Could you check a few things on this drawing? It's one solid part, dimensions in mm from its lowest x, y, z. A direction names the side the tool comes from. Give positions to 0.01 mm unless a question says otherwise; leave off trailing zeros. Order: outer loops, then holes, each group sorted by start corner. A loop starts at its lowest first (then second) coordinate and runs counter-clockwise, first axis right, second up. Notation, with made-up numbers: M 68,17.25 L 111,17.25 A25 cw 111,50.25 Z; hole C 67,80 d5. An arc over 180 degrees is marked long. Use one line per item in the form item = value. Start each with the question number.
1. I want a section at D-D, the plane x = 8.25. List the corners of the cut face in (y, z) for me, and give its area (3 significant figures).
2. Will these pins go through, and if not, where does the flat tip stop? P1, Ø3, axis at x = 6.5, y = 4, coming from the +Z side; P2, Ø4, axis at x = 7, z = 8, coming from the -Y side.
3. I want a section at A-A, the plane z = 6.5. List the corners of the cut face in (x, y) for me.
4. For the marked faces 4, 5, 6, 7 and 8, which set-ups out of +Z, -Z, +X, -X, +Y, -Y let a thin tool reach every point of the face, with its end or its side?
5. We'd pull the mould along Z, two halves only. Please class the marked faces 1, 2 and 3: +Z half, -Z half, draft (parallel to the pull), parting line (faces both ways), or undercut.
6. I need wall thicknesses on L1, parallel to X at y = 5.15, z = 6.5; L2, parallel to X at y = 2.3, z = 6.5; L3, parallel to Y at x = 9.25, z = 8.75. Which ranges of each line are inside material? Lowest first, please.
7. I want a section at C-C, the plane y = 5. List the corners of the cut face in (x, z) for me, and give its area (3 significant figures).
8. I want a section at B-B, the plane x = 6.5. List the corners of the cut face in (y, z) for me, and give its area (3 significant figures).
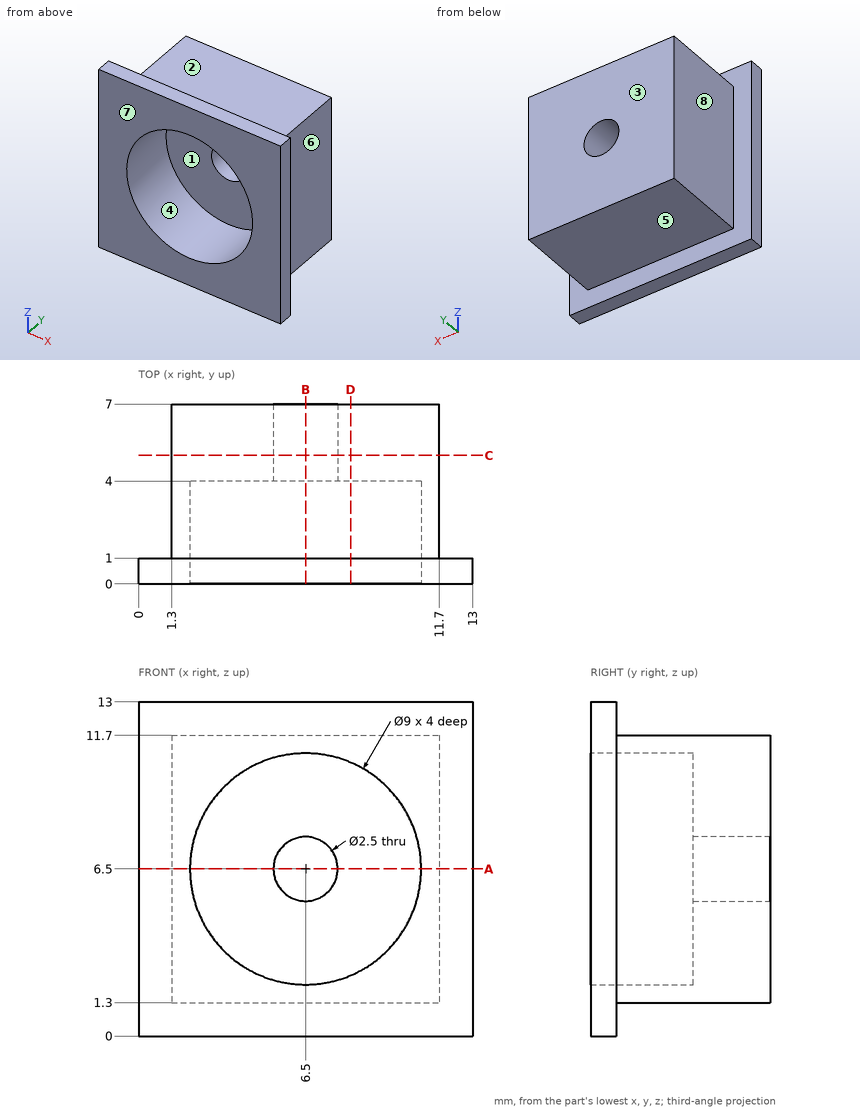
Check result:
q1.outline = M 0,0 L 1,0 L 1,1.3 L 7,1.3 L 7,11.7 L 1,11.7 L 1,13 L 0,13 L 0,10.65 L 4,10.65 L 4,2.35 L 0,2.35 Z
q1.area = 42.2 mm2
q2.P1 = 11.7
q2.P2 = 4
q3.outline = M 0,0 L 2,0 L 2,4 L 5.25,4 L 5.25,7 L 1.3,7 L 1.3,1 L 0,1 Z; M 7.75,4 L 11,4 L 11,0 L 13,0 L 13,1 L 11.7,1 L 11.7,7 L 7.75,7 Z
q4.face_4 = -Y
q4.face_5 = -Z, +X, -X, +Y
q4.face_6 = +Z, -Z, +X, +Y
q4.face_7 = +Z, -Z, +X, -X, -Y
q4.face_8 = +Z, -Z, -X, +Y
q5.face_1 = undercut
q5.face_2 = +Z half
q5.face_3 = draft
q6.L1 = 1.3 to 5.25, 7.75 to 11.7
q6.L2 = 1.3 to 2, 11 to 11.7
q6.L3 = 4 to 7
q7.outline = M 1.3,1.3 L 11.7,1.3 L 11.7,11.7 L 1.3,11.7 Z; hole C 6.5,6.5 d2.5
q7.area = 103 mm2
q8.outline = M 0,0 L 1,0 L 1,1.3 L 7,1.3 L 7,5.25 L 4,5.25 L 4,2 L 0,2 Z; M 0,11 L 4,11 L 4,7.75 L 7,7.75 L 7,11.7 L 1,11.7 L 1,13 L 0,13 Z
q8.area = 31.9 mm2
